Job drawing, mm, ordinate dimensions from the low corner. One solid piece. A direction names the side the tool comes from. Give positions to 0.01 mm unless a question says otherwise; leave off trailing zeros. Order: outer loops, then holes, each group sorted by start corner. A loop starts at its lowest first (then second) coordinate and runs counter-clockwise, first axis right, second up. Notation, with made-up numbers: (23.5, 18.25) -> (73.5, 18.25) arc R18 cw to (73.5, 42.25) -> close; hole circle Ø9 at (77.25, 9.5). An arc over 180 degrees is marked (long way). Use CSV: the item, a comma, the result in double quotes. Start each with the question number.
1. Cut at B-B on z = 2.1. List the corners of the cut face in (x, y) (1 decimal).
2. Cut at D-D on x = 2.25. List the corners of the cut face in (y, z).
3. Drop flat-ended pins along their axis: pin 1 (2 mm diameter, centred on x = 11.5, z = 4.5, fed in from +Y); pin 2 (2 mm diameter, centred on x = 4.5, y = 2, fed in from +Z); pin 3 (1.5 mm diameter, centred on x = 2, z = 4, fed in from -Y). Give the stop position or say it passes through.
4. Cut at C-C on x = 4.5. List the corners of the cut face in (y, z).
5. Cut at A-A on y = 2.75. List the corners of the cut face in (x, z), then the cut area to 3 significant figures.
6. Wall check: line 1 (X direction, y = 1.4, z = 4.3); line 2 (Y direction, x = 4.25, z = 2.65); line 3 (X direction, y = 3.8, z = 2.6). Give the ranges that are in metal, low to high. Write a range as from..to.
7. Pull direction Y, two halves, no side cores. Call the marked faces 4, 5 and 6: released by +Y, released by -Y, zero draft, split by the parting line, or undercut.
8. 3-axis set-ups, long thin cutter, end or side, ignore diameter. For the marked faces 1, 2 and 3: which of +Z, -Z, +X, -X, +Y, -Y reach the whole face in a straight line?
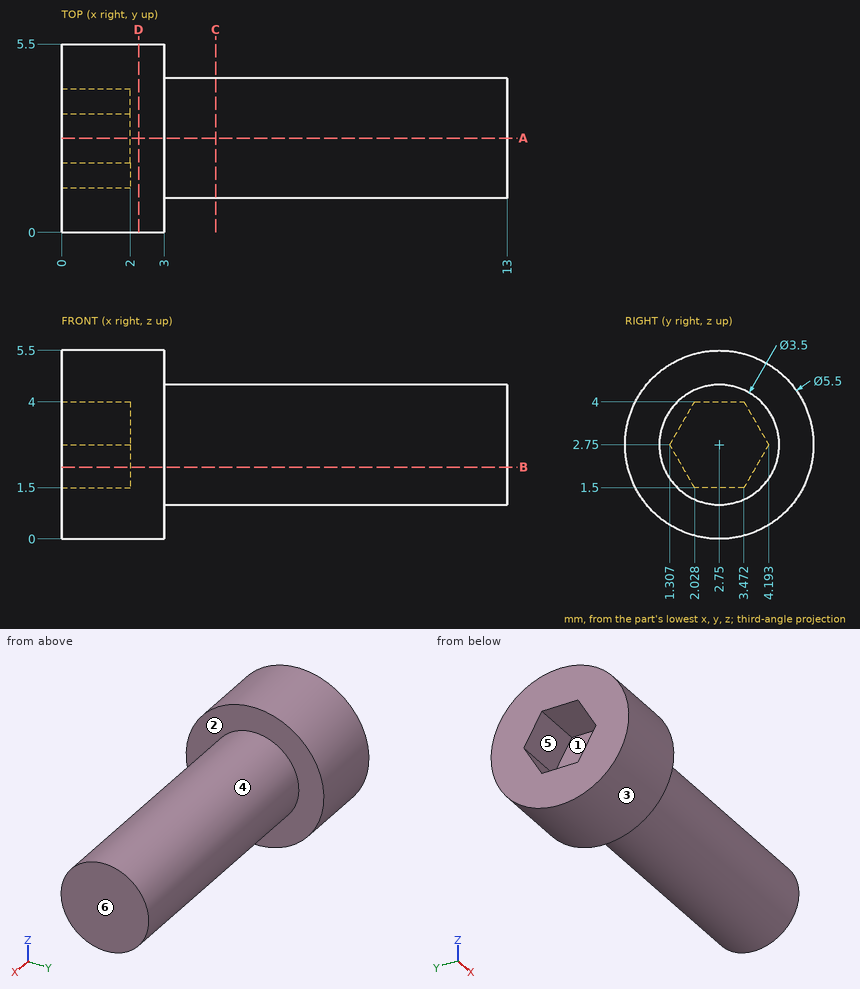
Verdict:
1,outline,"(0, 0.1) -> (3, 0.1) -> (3, 1.1) -> (13, 1.1) -> (13, 4.4) -> (3, 4.4) -> (3, 5.4) -> (0, 5.4) -> (0, 3.8) -> (2, 3.8) -> (2, 1.7) -> (0, 1.7) -> close"
2,outline,"circle Ø5.5 at (2.75, 2.75)"
3,pin 1,"y = 4.33"
3,pin 2,"z = 4.5"
3,pin 3,"y = 0.05"
4,outline,"circle Ø3.5 at (2.75, 2.75)"
5,outline,"(0, 0) -> (3, 0) -> (3, 1) -> (13, 1) -> (13, 4.5) -> (3, 4.5) -> (3, 5.5) -> (0, 5.5) -> (0, 4) -> (2, 4) -> (2, 1.5) -> (0, 1.5) -> close"
5,area,"46.5 mm^2"
6,line 1,"0..3"
6,line 2,"1..4.5"
6,line 3,"2..13"
7,face 4,"split by the parting line"
7,face 5,"undercut"
7,face 6,"zero draft"
8,face 1,"-X"
8,face 2,"+X"
8,face 3,"+X, -X"
